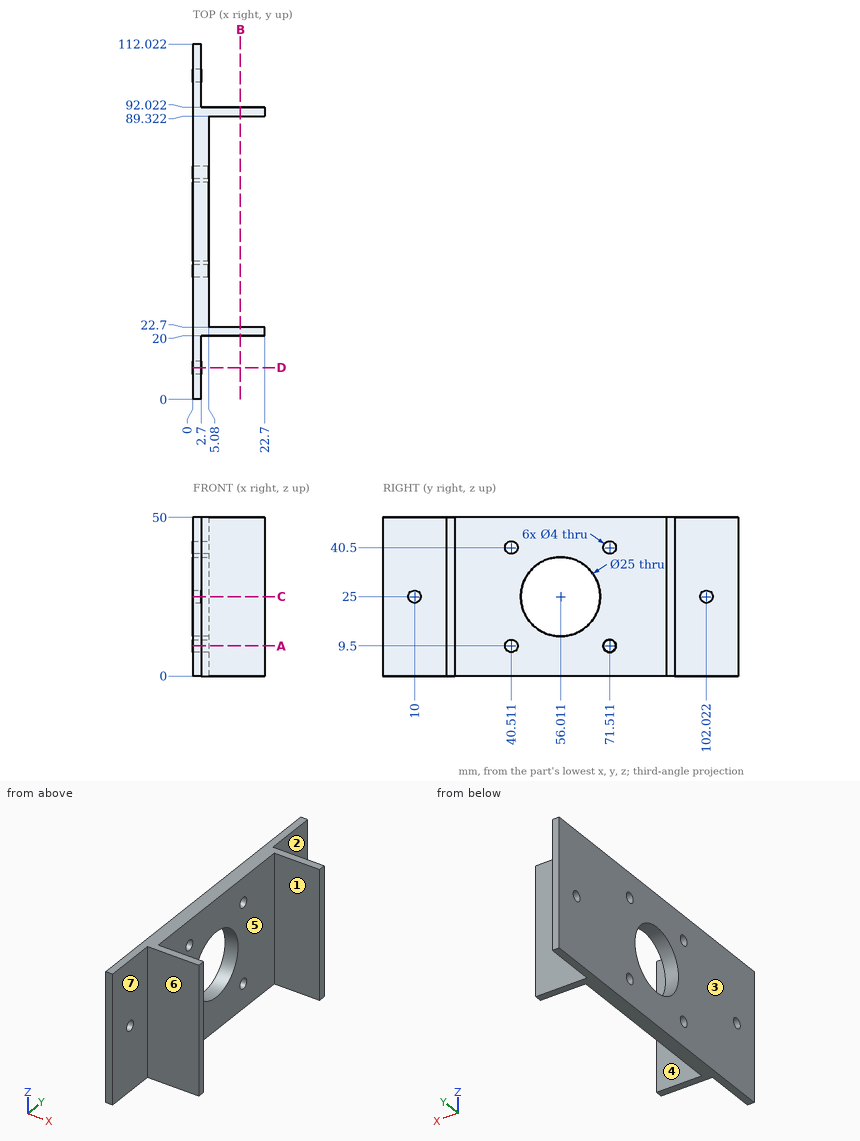
Verification items for this drawing (mm, ordinates from the low corner). A direction names the side the tool comes from. Give positions to 0.01 mm unless a question says otherwise; leave off trailing zeros. Write each loop counter-clockwise with the first axis right and the second up, starting at its lowest first coordinate (ties: lowest second). Pieces come first, ordered by that corner, then holes. Notation, with made-up numbers: (81, -1.75) -> (87, -1.75) arc R24 ccw to (87, 35.25) -> close; hole circle Ø8 at (14.5, 29). An arc over 180 degrees is marked (long way). Use CSV: the item, a comma, the result in double quotes. Start each with the question number.
Q1. Cross-section at C-C on z = 25. Enter the section's corners in (x, y).
Q2. Tool access check on the marked faces 1, 2 and 3. Record the directions out of +Z, -Z, +X, -X, +Y, -Y that give a thin tool (end or side, any length) a straight path to the whole face; none if there is none.
Q3. Depth check by flat-ended pin: P1, Ø1, axis at x = 14.5, z = 38, coming from the +Y side; P2, Ø10, axis at y = 81.5, z = 16, coming from the +X side; P3, Ø9, axis at x = 14, z = 14, coming from the -Y side. Enter the tip coordinate at first touch or a pass-through.
Q4. Cross-section at B-B on x = 15. Enter the section's corners in (y, z).
Q5. Release check for a two-part mould opening along Y. For the marked faces 4, 5, 6 and 7 record: +Y half, -Y half, draft (parallel to the pull), parting line (faces both ways), or undercut.
Q6. Scan lines: line 1 along Y through (x, z) = (1, 25); line 2 along Y through (x, z) = (1.4, 9.5); line 3 along Y through (x, z) = (11, 29.5). Record each from-to range of solid material in increasing order.
Q7. Cross-section at A-A on z = 9.5. Enter the section's corners in (x, y).
Q8. Cross-section at D-D on y = 10. Enter the section's corners in (x, z), and give its area (3 significant figures).
Working result:
1,outline,"(0, 0) -> (2.7, 0) -> (2.7, 8) -> (0, 8) -> close; (0, 12) -> (2.7, 12) -> (2.7, 20) -> (22.7, 20) -> (22.7, 22.7) -> (5.08, 22.7) -> (5.08, 43.51) -> (0, 43.51) -> close; (0, 68.51) -> (5.08, 68.51) -> (5.08, 89.32) -> (22.7, 89.32) -> (22.7, 92.02) -> (2.7, 92.02) -> (2.7, 100.02) -> (0, 100.02) -> close; (0, 104.02) -> (2.7, 104.02) -> (2.7, 112.02) -> (0, 112.02) -> close"
2,face 1,"+Z, -Z, +X"
2,face 2,"+Z, -Z, +X, +Y"
2,face 3,"+Z, -Z, -X, +Y, -Y"
3,P1,"stops at y = 92.02"
3,P2,"stops at x = 5.08"
3,P3,"stops at y = 20"
4,outline,"(20, 0) -> (22.7, 0) -> (22.7, 50) -> (20, 50) -> close; (89.32, 0) -> (92.02, 0) -> (92.02, 50) -> (89.32, 50) -> close"
5,face 4,"undercut"
5,face 5,"undercut"
5,face 6,"-Y half"
5,face 7,"draft"
6,line 1,"y = 0 to 8, 12 to 43.51, 68.51 to 100.02, 104.02 to 112.02"
6,line 2,"y = 0 to 38.51, 42.51 to 69.51, 73.51 to 112.02"
6,line 3,"y = 20 to 22.7, 89.32 to 92.02"
7,outline,"(0, 0) -> (2.7, 0) -> (2.7, 20) -> (22.7, 20) -> (22.7, 22.7) -> (5.08, 22.7) -> (5.08, 38.51) -> (0, 38.51) -> close; (0, 42.51) -> (5.08, 42.51) -> (5.08, 69.51) -> (0, 69.51) -> close; (0, 73.51) -> (5.08, 73.51) -> (5.08, 89.32) -> (22.7, 89.32) -> (22.7, 92.02) -> (2.7, 92.02) -> (2.7, 112.02) -> (0, 112.02) -> close"
8,outline,"(0, 0) -> (2.7, 0) -> (2.7, 23) -> (0, 23) -> close; (0, 27) -> (2.7, 27) -> (2.7, 50) -> (0, 50) -> close"
8,area,"124 mm^2"
